```python
from build123d import *

# Parameters (mm, degrees)
PAD024_DEPTH      = 4
PAD024_DEPTH_BACK = 4
SKETCH047_R       = 1.3
POCKET_DEPTH      = 20.001
SKETCH048_R       = 1.3
POCKET001_DEPTH   = 20.001


with BuildPart() as part:
    # Sketch046 → Pad024 (new body, two sides)
    with BuildSketch(Plane(origin=(118.5, -33.5, -4.5), x_dir=(-1, 0, 0), z_dir=(0, 1, 0))) as pad024_sk:
        Polygon((0, 0), (20, 0), (20, -7.5), (7.5, -20), (0, -20), align=None)
    extrude(amount=PAD024_DEPTH)
    extrude(pad024_sk.sketch, amount=-PAD024_DEPTH_BACK)

    # Sketch047 → Pocket (cut, through all)
    with BuildSketch(Plane(origin=(118.5, -33.5, -4.5), x_dir=(0, 0, -1), z_dir=(1, 0, 0))):
        with Locations((12, 0)):
            Circle(SKETCH047_R)
    extrude(amount=-POCKET_DEPTH, mode=Mode.SUBTRACT)

    # Sketch048 → Pocket001 (cut, through all)
    with BuildSketch(Plane(origin=(118.5, -33.5, -4.5), x_dir=(1, 0, 0), z_dir=(0, 0, 1))):
        with Locations((-12, 0)):
            Circle(SKETCH048_R)
    extrude(amount=-POCKET001_DEPTH, mode=Mode.SUBTRACT)


solid = part.part
```
The model under review builds one solid part; all positions refer to its coordinate system, in mm. Round coordinates to 2 decimals unless told otherwise and drop trailing zeros. Order: outer loops, then holes, each group sorted by start corner. A loop starts at its lowest first (then second) coordinate and runs counter-clockwise, first axis right, second up. Notation, with made-up numbers: (79.5, 82.25) - (117.5, 82.25) arc R9 ccw to (117.5, 93.25) - close; hole circle Ø9 at (54.25, 30.25). An arc over 180 degrees is marked (long way). Answer in a Markdown table with one row per item.
(1) Take a section at B-B on z = -9.5. Write out the cut boundary in (x, y), plus the area to 3 significant figures.
Result set:
| item | result |
|---|---|
| outline | (98.5, -37.5) - (118.5, -37.5) - (118.5, -29.5) - (98.5, -29.5) - close; hole circle Ø2.6 at (106.5, -33.5) |
| area | 155 mm2 |
(2) Take a section at D-D on y = -36.25. Write out the cut boundary in (x, z).
Result set:
| item | result |
|---|---|
| outline | (98.5, -12) - (111, -24.5) - (118.5, -24.5) - (118.5, -4.5) - (98.5, -4.5) - close |
(3) Take a section at C-C on x = 112. Write out the cut boundary in (y, z), plus the area to 3 significant figures.
Result set:
| item | result |
|---|---|
| outline | (-37.5, -24.5) - (-29.5, -24.5) - (-29.5, -4.5) - (-37.5, -4.5) - close; hole circle Ø2.6 at (-33.5, -16.5) |
| area | 155 mm2 |
(4) Clearance check with flat-ended pins moving along their axes: P1, Ø3.5, axis at y = -33.5, z = -16.5, coming from the -X side; P2, Ø4, axis at y = -33.5, z = -16.5, coming from the -X side; P3, Ø1, axis at y = -36, z = -20, coming from the -X side; P4, Ø2, axis at x = 106.5, y = -33.5, coming from the -Z side. State where each tip first meets the part, or that it passes through.
Result set:
| item | result |
|---|---|
| P1 | stops at x = 101.25 |
| P2 | stops at x = 101 |
| P3 | stops at x = 106 |
| P4 | passes through |
(5) Take a section at A-A on y = -33.5. Write out the cut boundary in (x, z).
Result set:
| item | result |
|---|---|
| outline | (98.5, -12) - (101.7, -15.2) - (105.2, -15.2) - (105.2, -4.5) - (98.5, -4.5) - close; (104.3, -17.8) - (105.2, -18.7) - (105.2, -17.8) - close; (107.8, -21.3) - (111, -24.5) - (118.5, -24.5) - (118.5, -17.8) - (107.8, -17.8) - close; (107.8, -15.2) - (118.5, -15.2) - (118.5, -4.5) - (107.8, -4.5) - close |
(6) For line 1 (Y direction, x = 104.2, z = -16.5); line 2 (X direction, y = -33.5, z = -8.75); line 3 (Z direction, x = 116.5, y = -32.75), list the stretches that pass through material, from the lowest coordinate up. Write a range as from..to.
Result set:
| item | result |
|---|---|
| line 1 | y = -37.5..-34.8, -32.2..-29.5 |
| line 2 | x = 98.5..105.2, 107.8..118.5 |
| line 3 | z = -24.5..-17.56, -15.44..-4.5 |
(7) Mouldability with a two-part tool opening along Y and no side actions: class faces 1 (the face through (115, -33, -24.5)), 2 (the face through (111, -37.5, -12)), 3 (the face through (112.58, -33.11, -17.74)) as released by +Y, released by -Y, zero draft, split by the parting line, or undercut.
Result set:
| item | result |
|---|---|
| face 1 | zero draft |
| face 2 | released by -Y |
| face 3 | undercut |
